from build123d import *

# Parameters (mm, degrees)
BOSS_EXTRUDE1_DEPTH      = 800
BOSS_EXTRUDE2_DEPTH      = 50
BOSS_EXTRUDE2_DEPTH_BACK = 850
SKETCH2_W                = 370
SKETCH2_H                = 80


with BuildPart() as part:
    # Sketch1 → Boss-Extrude1 (new body)
    with BuildSketch(Plane(origin=(0, 0, 0), x_dir=(1, 0, 0), z_dir=(0, 1, 0))):
        Polygon((-228, 90), (-260, 90), (-260, 0), (0, 0), (0, 90), (-32, 90), (-32, 81), (-24, 81), (-24, 72), (-56, 72), (-56, 81), (-48, 81), (-48, 90), (-122, 90), (-122, 81), (-114, 81), (-114, 72), (-146, 72), (-146, 81), (-138, 81), (-138, 90), (-212, 90), (-212, 81), (-204, 81), (-204, 72), (-236, 72), (-236, 81), (-228, 81), align=None)
    extrude(amount=BOSS_EXTRUDE1_DEPTH)

    # Sketch2 → Boss-Extrude2 (add, two sides: drawn at the far end of the back side and taken through both)
    with BuildSketch(Plane.XZ.offset(-BOSS_EXTRUDE2_DEPTH_BACK)):
        with Locations((-153, 6)):
            Rectangle(SKETCH2_W, SKETCH2_H)
    extrude(amount=BOSS_EXTRUDE2_DEPTH + BOSS_EXTRUDE2_DEPTH_BACK)


solid = part.part
Verification items for the finished model (mm, model axes). A direction names the side the tool comes from. Give positions to 0.01 mm unless a question says otherwise; leave off trailing zeros. Write each loop counter-clockwise with the first axis right and the second up, starting at its lowest first coordinate (ties: lowest second). Pieces come first, ordered by that corner, then holes. Notation, with made-up numbers: M -9,54.5 L 18,54.5 A14 cw 18,62.5 Z; hole C 77.5,7 d8. An arc over 180 degrees is marked long. Write item = value, one per line.
(1) Go/stop test with flat-tipped pins: pin 1 Ø4.5 at (y, z) = (224.5, -75) entering from +X; pin 2 Ø8 at (x, z) = (-168, -69) entering from -Y; pin 3 Ø10 at (y, z) = (467, -84) entering from -X. Record where each tip stops, or that it passes through.
Found:
pin_1 = 0
pin_2 = 0
pin_3 = -260
(2) Sectioned sample at B-B (x = -102). Record the cut outline in (y, z), then the cut area to 3 significant figures.
Found:
outline = M -50,-34 L 0,-34 L 0,-90 L 800,-90 L 800,-34 L 850,-34 L 850,46 L -50,46 Z
area = 117,000 mm2
(3) Access from +Z, -Z, +X, -X, +Y, -Y to the whole of each face (thin tool, end or side, straight path). Record for faces 4 (the face through (0, 394, -62)), 5 (the face through (-244, 394, -90)), 6 (the face through (-130, 394, -72)), 7 (the face through (-132, 0, -62)), 8 (the face through (-132, 800, -62)).
Found:
face_4 = -Z, +X, +Y, -Y
face_5 = -Z, +X, -X, +Y, -Y
face_6 = +Y, -Y
face_7 = -Z, +X, -X, -Y
face_8 = -Z, +X, -X, +Y
(4) Material ranges on line 1 (Z direction, x = -119.5, y = 241.5); line 2 (Z direction, x = 9, y = 532.5); line 3 (Z direction, x = -215, y = 777), recorded low to high.
Found:
line_1 = -90 to -81, -72 to 46
line_2 = -34 to 46
line_3 = -72 to 46
(5) Draft check along X on faces 1 (the face through (-220, 394, -72)), 2 (the face through (-260, 394, -62)), 3 (the face through (-16, 394, -90)). Enter one of: released by +X, released by -X, zero draft, split by the parting line, or undercut.
Found:
face_1 = undercut
face_2 = released by -X
face_3 = zero draft
(6) Sectioned sample at C-C (x = -271). Record the cut outline in (y, z), then the cut area to 3 significant figures.
Found:
outline = M -50,-34 L 850,-34 L 850,46 L -50,46 Z
area = 72,000 mm2
